Geometry: final body of the model. Coordinates: model frame, mm. Round coordinates to 2 decimals unless told otherwise and drop trailing zeros. Write each loop counter-clockwise with the first axis right and the second up, starting at its lowest first coordinate (ties: lowest second). Pieces come first, ordered by that corner, then holes. Notation, with made-up numbers: M 58,-18 L 88,-18 A30 cw 88,4 Z; hole C -8.5,38 d4. An arc over 180 degrees is marked long. Use one line per item in the form item = value. Start each with the question number.
Item 1: Section query C-C (z = 108). Return loops of the section in (x, y).
Item 2: Ray query, probe 1 along Y at (x, z) = (4.75, 35); probe 2 along Y at (x, z) = (2.75, 152); probe 3 along Z at (x, y) = (6.25, 12). Return the intervals inside material, ascending.
Item 3: Section query A-A (y = -13). Return loops of the section in (x, z), and give its area (3 significant figures).
Item 4: Section query D-D (y = -20). Return loops of the section in (x, z).
Item 5: Pin query (flat end, axial travel): pin 1 Ø3 at (x, z) = (5, 73.5) entering from -Y; pin 2 Ø1.9 at (x, z) = (2, 13.5) entering from -Y; pin 3 Ø3 at (x, z) = (3, 69.5) entering from +Y; pin 4 Ø6 at (y, z) = (5, 70) entering from -X. Return the tip coordinate at first contact, or that it passes through.
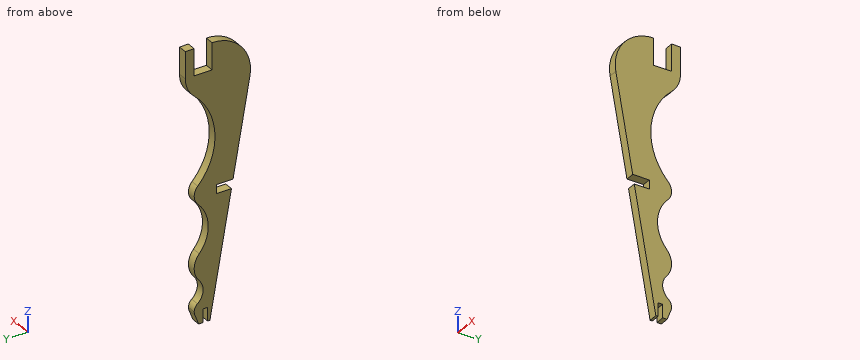
from build123d import *

# Parameters (mm, degrees)
BOSS_EXTRUDE1_DEPTH = 6.35
SKETCH2_W           = 6.35
SKETCH2_H           = 11.789754461
CUT_EXTRUDE1_DEPTH  = 206.585562738
CUT_EXTRUDE2_DEPTH  = 206.585562738


with BuildPart() as part:
    # Sketch1 → Boss-Extrude1 (new body)
    with BuildSketch(Plane(origin=(0, 0, 0), x_dir=(0, 0, -1), z_dir=(1, 0, 0))):
        with BuildLine():
            Line((-19.05, 0), (-19.05, 3.175))
            Line((-19.05, 3.175), (0, 3.175))
            Line((0, 3.175), (0, 9.525))
            Line((0, 9.525), (-19.05, 9.525))
            ThreePointArc((-19.05, 9.525), (-21.772170288, 8.911923298), (-23.968703037, 7.191075252))
            ThreePointArc((-23.968703037, 7.191075252), (-31.563196652, 3.209635371), (-39.693056937, 5.936092509))
            ThreePointArc((-39.693056937, 5.936092509), (-49.128661086, 9.524999891), (-58.565155627, 5.938434313))
            ThreePointArc((-58.565155627, 5.938434313), (-76.175633399, -0.485223061), (-93.413507935, 6.880099943))
            ThreePointArc((-93.413507935, 6.880099943), (-99.75616874, 9.524590732), (-106.147751964, 7.000637182))
            ThreePointArc((-106.147751964, 7.000637182), (-138.580790239, -5.246129508), (-169.944766377, 9.525))
            ThreePointArc((-169.944766377, 9.525), (-176.370039167, 14.215248831), (-184.15, 15.875))
            Line((-184.15, 15.875), (-203.2, 15.875))
            Line((-203.2, 15.875), (-203.2, 9.525))
            Line((-203.2, 9.525), (-184.15, 9.525))
            Line((-184.15, 9.525), (-184.15, -3.175))
            Line((-184.15, -3.175), (-203.2, -3.175))
            ThreePointArc((-203.2, -3.175), (-193.412202449, -24.164999585), (-171.041454914, -30.159223321))
            Line((-171.041454914, -30.159223321), (-9.525, -1.679514491))
            Line((-9.525, -1.679514491), (-9.525, 0))
            Line((-9.525, 0), (-19.05, 0))
        make_face()
    extrude(amount=BOSS_EXTRUDE1_DEPTH)

    # Sketch2 → Cut-Extrude1 (cut, through all)
    with BuildSketch(Plane(origin=(6.35, 0, 0), x_dir=(0, 0, -1), z_dir=(1, 0, 0))):
        with Locations((-99.700659688, -12.244877231)):
            Rectangle(SKETCH2_W, SKETCH2_H)
    extrude(amount=-CUT_EXTRUDE1_DEPTH, mode=Mode.SUBTRACT)

    # Sketch3 → Cut-Extrude2 (cut, through all)
    with BuildSketch(Plane(origin=(6.35, 0, 0), x_dir=(0, 0, -1), z_dir=(1, 0, 0))):
        with BuildLine():
            Line((-9.525, 3.175), (-9.525, 6.35))
            Line((-9.525, 6.35), (-16.795425987, 9.11127796))
            ThreePointArc((-16.795425987, 9.11127796), (-17.903890286, 9.420713132), (-19.05, 9.525))
            Line((-19.05, 9.525), (0, 9.525))
            Line((0, 9.525), (0, 3.175))
            Line((0, 3.175), (-9.525, 3.175))
        make_face()
    extrude(amount=-CUT_EXTRUDE2_DEPTH, mode=Mode.SUBTRACT)


solid = part.part
Working result:
q1.outline = M 0,-19.04 L 6.35,-19.04 L 6.35,5.33 L 0,5.33 Z
q2.probe_1 = -6.17 to 3.48
q2.probe_2 = -26.8 to -2.61
q2.probe_3 = 172.63 to 203.2
q3.outline = M 0,73.73 L 6.35,73.73 L 6.35,96.53 L 0,96.53 Z; M 0,102.88 L 6.35,102.88 L 6.35,201.38 L 0,201.38 Z
q3.area = 770 mm²
q4.outline = M 0,113.43 L 6.35,113.43 L 6.35,197.43 L 0,197.43 Z
q5.pin_1 = -13.22
q5.pin_2 = -2.55
q5.pin_3 = 0.63
q5.pin_4 = through
